Input: part model. Units: mm. Frame: model coordinates. A direction names the side the tool comes from. Give positions to 0.01 mm unless a question says otherwise; leave off trailing zeros. Loops run counter-clockwise (first coordinate to the right, second up) from the corner with the lowest first, then second, coordinate; pieces in that order, holes last. Notation, with made-up numbers: M 41.25,-14.5 L 88.25,-14.5 A16 cw 88.25,2.5 Z; hole C 18.5,-3.5 d8. An arc over 180 degrees is marked long. Answer as a JSON object with one key per item and string values. Group by question number.
1) First-contact query: P1, Ø10, axis at x = -2, z = 2.5, coming from the +Y side; P2, Ø1, axis at y = 2.5, z = 4.5, coming from the +X side; P3, Ø1, axis at x = 8, y = 1, coming from the +Z side; P4, Ø3, axis at y = -1, z = -6, coming from the +X side. Flat tips, straight axial feed; report the tip coordinate or a pass-through.
2) Section query D-D on z = 8.75. Return loops of the section in (x, y), plus the area to 3 significant figures.
3) Section query A-A on z = 0. Return loops of the section in (x, y).
4) Ray query, L1, parallel to Z at x = 0, y = 3.35; L2, parallel to Z at x = 0, y = 1; L3, parallel to Y at x = 7.5, z = -1. Return the intervals inside material, ascending.
5) Draft query along Z for faces 4 (the cylindrical face through (5.919, -0.05, 9.284)), 5 (the flat face through (3, 3.581, -10)), 6 (the flat face through (4.4, -3.2, -4.4)). Return one class per face: +Z half, -Z half, draft (parallel to the pull), parting line (faces both ways), or undercut.
6) Access query for faces 1 (the cylindrical face through (-0.78, -3.39, 5.93)), 2 (the cylindrical face through (3.852, 0.05, 1.213)), 3 (the cylindrical face through (-1.323, 3.394, 10.074)). Directions: +Z, -Z, +X, -X, +Y, -Y. A direction counts if a zero-diameter tool reaches every point of the face in a straight line with its end or side. Return the directions, or none.
7) Section query B-B on x = 0. Return loops of the section in (y, z), plus the area to 3 significant figures.
8) Section query C-C on y = 2.5. Return loops of the section in (x, z).
from build123d import *

# Parameters (mm, degrees)
F0_R     = 11.0109
F0_R_2   = 5.969
F1_DEPTH = 3.5814
F2_R     = 10.16
F2_R_2   = 5.9817
F3_DEPTH = 0.381
F4_R     = 5.969
F4_R_2   = 4.0386
F5_DEPTH = 3.5814


# Not quite as in the source:
# - a pattern or mirror of a feature is missing from the dataset's text; its kind, count and spacing are read off the source's solid


with BuildPart() as f1:
    # F0 (on Front) → F1 (new body, symmetric)
    with BuildSketch(Plane.XZ):
        Circle(F0_R)
        Circle(F0_R_2, mode=Mode.SUBTRACT)
    extrude(amount=F1_DEPTH, both=True)

    # F2 (on face) → F3 (cut)
    with BuildSketch(Plane.XZ.offset(3.5814)):
        Circle(F2_R)
        Circle(F2_R_2, mode=Mode.SUBTRACT)
    f3 = extrude(amount=-F3_DEPTH, mode=Mode.SUBTRACT)

    # F3_copies: F3 across plane
    add(f3.mirror(Plane.ZX), mode=Mode.SUBTRACT)

    # F4 (on Front) → F5 (join, symmetric)
    with BuildSketch(Plane.XZ):
        Circle(F4_R)
        Circle(F4_R_2, mode=Mode.SUBTRACT)
    extrude(amount=F5_DEPTH, both=True)


solid = f1.part
Output:
{
 "1": {"P1": "stops at y = 3.58", "P2": "stops at x = 10.26", "P3": "stops at z = 8.06", "P4": "stops at x = 10.05"},
 "2": {"outline": "M -6.68,-3.58 L -5.16,-3.58 L -5.16,-3.2 L 5.16,-3.2 L 5.16,-3.58 L 6.68,-3.58 L 6.68,3.58 L 5.16,3.58 L 5.16,3.2 L -5.16,3.2 L -5.16,3.58 L -6.68,3.58 Z", "area": "87.9 mm^2"},
 "3": {"outline": "M -11.01,-3.58 L -10.16,-3.58 L -10.16,-3.2 L -5.98,-3.2 L -5.98,-3.58 L -4.04,-3.58 L -4.04,3.58 L -5.98,3.58 L -5.98,3.2 L -10.16,3.2 L -10.16,3.58 L -11.01,3.58 Z; M 4.04,-3.58 L 5.98,-3.58 L 5.98,-3.2 L 10.16,-3.2 L 10.16,-3.58 L 11.01,-3.58 L 11.01,3.58 L 10.16,3.58 L 10.16,3.2 L 5.98,3.2 L 5.98,3.58 L 4.04,3.58 Z"},
 "4": {"L1": "z = -11.01 to -10.16, -5.98 to -4.04, 4.04 to 5.98, 10.16 to 11.01", "L2": "z = -11.01 to -4.04, 4.04 to 11.01", "L3": "y = -3.2 to 3.2"},
 "5": {"face 4": "parting line", "face 5": "draft", "face 6": "undercut"},
 "6": {"face 1": "-Y", "face 2": "+Y, -Y", "face 3": "+Y"},
 "7": {"outline": "M -3.58,-11.01 L 3.58,-11.01 L 3.58,-10.16 L 3.2,-10.16 L 3.2,-5.98 L 3.58,-5.98 L 3.58,-4.04 L -3.58,-4.04 L -3.58,-5.98 L -3.2,-5.98 L -3.2,-10.16 L -3.58,-10.16 Z; M -3.58,4.04 L 3.58,4.04 L 3.58,5.98 L 3.2,5.98 L 3.2,10.16 L 3.58,10.16 L 3.58,11.01 L -3.58,11.01 L -3.58,10.16 L -3.2,10.16 L -3.2,5.98 L -3.58,5.98 Z", "area": "93.5 mm^2"},
 "8": {"outline": "C 0,0 d22.02; hole C 0,0 d8.08"}
}
